```python
from build123d import *

# Parameters (mm, degrees)
BOSS_EXTRUDE1_DEPTH = 38.1
SKETCH5_R           = 2.4892
CUT_EXTRUDE1_DEPTH  = 51.899122045
SKETCH6_R           = 2.4892
CUT_EXTRUDE2_DEPTH  = 51.899122045


with BuildPart() as part:
    # Sketch2 → Boss-Extrude1 (new body)
    with BuildSketch(Plane.XY):
        Polygon((0, 0), (0, -25.4), (3.175, -25.4), (3.175, -3.175), (25.4, -3.175), (25.4, 0), align=None)
    extrude(amount=BOSS_EXTRUDE1_DEPTH)

    # Sketch5 → Cut-Extrude1 (cut, through all)
    with BuildSketch(Plane(origin=(3.175, 0, 0), x_dir=(0, 0, -1), z_dir=(1, 0, 0))):
        with Locations(Location((-6.35, -12.7, 0), (0, 0, 90))):
            Circle(SKETCH5_R)
        with Locations(Location((-19.05, -12.7, 0), (0, 0, 90))):
            Circle(SKETCH5_R)
        with Locations(Location((-31.75, -12.7, 0), (0, 0, 90))):
            Circle(SKETCH5_R)
        with Locations((-44.45, -12.7)):
            Circle(SKETCH5_R)
    extrude(amount=-CUT_EXTRUDE1_DEPTH, mode=Mode.SUBTRACT)

    # Sketch6 → Cut-Extrude2 (cut, through all)
    with BuildSketch(Plane.XZ.offset(3.175)):
        with Locations((12.7, 6.35)):
            Circle(SKETCH6_R)
        with Locations((12.7, 19.05)):
            Circle(SKETCH6_R)
        with Locations((12.7, 31.75)):
            Circle(SKETCH6_R)
        with Locations((12.7, 44.45)):
            Circle(SKETCH6_R)
    extrude(amount=-CUT_EXTRUDE2_DEPTH, mode=Mode.SUBTRACT)


solid = part.part
```
Here's how the part is built. I have some questions about the finished solid (model axes, mm). Coordinates: 2 decimals unless noted, no trailing zeros. Loops run counter-clockwise (first coordinate to the right, second up) from the corner with the lowest first, then second, coordinate; pieces in that order, holes last. Notation, with made-up numbers: (15, 40.5) - (41, 40.5) arc R5 cw to (41, 46.5) - close; hole circle Ø3 at (-39.75, 86.5). An arc over 180 degrees is marked (long way). Return JSON: item names as keys, results as strings. Group by question number.
Item 1: Will these pins go through, and if not, where does the flat tip stop? P1, Ø1, axis at y = -22, z = 29, coming from the +X side (3 decimals); P2, Ø6, axis at x = 22.5, z = 16, coming from the -Y side (3 decimals).
Item 2: We'd pull the mould along X, two halves only. Please class faces 1 (the face through (10.213, -1.61, 31.859)), 2 (the face through (17, -3.175, 19)), 3 (the face through (3.175, -17, 19)): +X half, -X half, draft (parallel to the pull), parting line (faces both ways), or undercut.
Item 3: If we section it at D-D on z = 8: Write out the boundary of the cut face in (x, y) (3 decimals), and give its area (3 significant figures).
Item 4: If we section it at B-B on x = 12.7: Write out the boundary of the cut face in (y, z) (3 decimals).
Item 5: I need wall thicknesses on line 1 (Z direction, x = 1.45, y = -12.7); line 2 (X direction, y = -20, z = 24) (3 decimals); line 3 (Y direction, x = 20.5, z = 21) (3 decimals). Which ranges of each line are inside material? Lowest first, please. Write a range as from..to.
Item 6: If we section it at A-A on z = 19.05: Write out the boundary of the cut face in (x, y) (3 decimals), and give its area (3 significant figures).
Item 7: If we section it at C-C on y = -12.7: Write out the boundary of the cut face in (x, z) (3 decimals).
Calculated:
{
 "1": {"P1": "stops at x = 3.175", "P2": "stops at y = -3.175"},
 "2": {"face 1": "undercut", "face 2": "draft", "face 3": "+X half"},
 "3": {"outline": "(0, -25.4) - (3.175, -25.4) - (3.175, -14.564) - (0, -14.564) - close; (0, -10.836) - (3.175, -10.836) - (3.175, -3.175) - (10.836, -3.175) - (10.836, 0) - (0, 0) - close; (14.564, -3.175) - (25.4, -3.175) - (25.4, 0) - (14.564, 0) - close", "area": "128 mm^2"},
 "4": {"outline": "(-3.175, 0) - (0, 0) - (0, 3.861) - (-3.175, 3.861) - close; (-3.175, 8.839) - (0, 8.839) - (0, 16.561) - (-3.175, 16.561) - close; (-3.175, 21.539) - (0, 21.539) - (0, 29.261) - (-3.175, 29.261) - close; (-3.175, 34.239) - (0, 34.239) - (0, 38.1) - (-3.175, 38.1) - close"},
 "5": {"line 1": "z = 0..3.86, 8.84..16.56, 21.54..29.26, 34.24..38.1", "line 2": "x = 0..3.175", "line 3": "y = -3.175..0"},
 "6": {"outline": "(0, -25.4) - (3.175, -25.4) - (3.175, -15.189) - (0, -15.189) - close; (0, -10.211) - (3.175, -10.211) - (3.175, -3.175) - (10.211, -3.175) - (10.211, 0) - (0, 0) - close; (15.189, -3.175) - (25.4, -3.175) - (25.4, 0) - (15.189, 0) - close", "area": "120 mm^2"},
 "7": {"outline": "(0, 0) - (3.175, 0) - (3.175, 3.861) - (0, 3.861) - close; (0, 8.839) - (3.175, 8.839) - (3.175, 16.561) - (0, 16.561) - close; (0, 21.539) - (3.175, 21.539) - (3.175, 29.261) - (0, 29.261) - close; (0, 34.239) - (3.175, 34.239) - (3.175, 38.1) - (0, 38.1) - close"}
}
